Read the model definition and answer for the solid it produces. Units are mm, in the model's axes. Face numbers are marked on the shaded views. A direction names the side the tool comes from. Round coordinates to 2 decimals unless told otherwise and drop trailing zeros. Order: outer loops, then holes, each group sorted by start corner. A loop starts at its lowest first (then second) coordinate and runs counter-clockwise, first axis right, second up. Notation, with made-up numbers: (75, -14) -> (111, -14) arc R21 cw to (111, 16) -> close; hole circle Ø10 at (35.25, 19). An arc over 180 degrees is marked (long way). One line per item, written item: value. Start each with the question number.
1. For the marked faces 1 and 2, determine the directions among +Z, -Z, +X, -X, +Y, -Y from which every point of the face is accessible in a straight line to the end or side of a thin tool.
2. Consider line 1 (Y direction, x = -430, z = 108.5); line 2 (X direction, y = 2, z = 186.5); line 3 (Z direction, x = -398, y = -403.5). Determine where each line is inside the solid, lowest interval first.
3. Section C-C (x = -496.5) is taken. Give the vertices of the cut face in (y, z).
4. The mould has two halves that part along Y. Classify the marked faces 3, 4 and 5: released by +Y, released by -Y, zero draft, split by the parting line, or undercut.
5. Section A-A (z = 169) is taken. Give the vertices of the cut face in (x, y), then the cut area to 3 significant figures.
6. Section B-B (y = -279) is taken. Give the vertices of the cut face in (x, z), then the cut area to 3 significant figures.
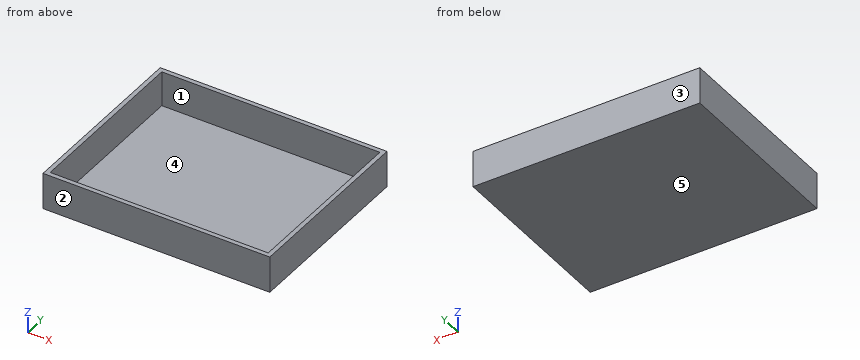
from build123d import *

# Parameters (mm, degrees)
F0_W     = 1560
F0_H     = 1260
F0_W_2   = 1500
F0_H_2   = 1200
F1_DEPTH = 250
F2_DEPTH = 10


with BuildPart() as f1:
    # F0 (on Top) → F1 (new body)
    with BuildSketch(Plane.XY):
        Rectangle(F0_W, F0_H)
        Rectangle(F0_W_2, F0_H_2, mode=Mode.SUBTRACT)
    extrude(amount=F1_DEPTH)

    # F0 (on Top) → F2 (join)
    with BuildSketch(Plane.XY):
        Rectangle(F0_W, F0_H)
        Rectangle(F0_W_2, F0_H_2, mode=Mode.SUBTRACT)
        Rectangle(F0_W_2, F0_H_2)
    extrude(amount=F2_DEPTH)


solid = f1.part
Answer:
1. face 1: +Z
1. face 2: +Z, -Z, +X, -X, -Y
2. line 1: -630 to -600, 600 to 630
2. line 2: -780 to -750, 750 to 780
2. line 3: 0 to 10
3. outline: (-630, 0) -> (630, 0) -> (630, 250) -> (600, 250) -> (600, 10) -> (-600, 10) -> (-600, 250) -> (-630, 250) -> close
4. face 3: released by +Y
4. face 4: undercut
4. face 5: zero draft
5. outline: (-780, -630) -> (780, -630) -> (780, 630) -> (-780, 630) -> close; hole (-750, -600) -> (750, -600) -> (750, 600) -> (-750, 600) -> close
5. area: 166,000 mm^2
6. outline: (-780, 0) -> (780, 0) -> (780, 250) -> (750, 250) -> (750, 10) -> (-750, 10) -> (-750, 250) -> (-780, 250) -> close
6. area: 30,000 mm^2
